```python
from build123d import *

# Parameters (mm, degrees)
F0_W          = 46
F0_H          = 58
F1_DEPTH      = 6
F2_W          = 38
F2_H          = 38
F3_DEPTH      = 3
F4_W          = 33
F4_H          = 33
F5_DEPTH      = 3.001
F6_W          = 26
F6_H          = 5
F7_DEPTH      = 3.001
F7_DEPTH_BACK = 3.001
F8_W          = 26
F8_H          = 5
F9_DEPTH      = 3.001
F9_DEPTH_BACK = 3.001
F10_SIZE      = 3
F11_W         = 4.5
F11_H         = 20
F12_DEPTH     = 46
F13_W         = 4
F13_H         = 9.5
F14_DEPTH     = 10
F15_T4_DEPTH  = 4
F16_W         = 4
F16_H         = 9.5
F17_DEPTH     = 10
F18_T4_DEPTH  = 4
F19_R         = 2
F20_DEPTH     = 4.501


# Not quite as in the source:
# - a fillet or chamfer that OpenCascade refuses, or shapes differently, is made with other operations: its cross-section is extruded or revolved along the edge and cut away or added


with BuildPart() as f1:
    # F0 (on Top) → F1 (new body)
    with BuildSketch(Plane.XY):
        Rectangle(F0_W, F0_H)
    extrude(amount=F1_DEPTH)

    # F2 (on face) → F3 (cut)
    with BuildSketch(Plane.XY.offset(6)):
        with Locations((0, 4)):
            Rectangle(F2_W, F2_H)
    extrude(amount=-F3_DEPTH, mode=Mode.SUBTRACT)

    # F4 (on face) → F5 (cut, through all)
    with BuildSketch(Plane.XY.offset(3)):
        with Locations((0, 4)):
            Rectangle(F4_W, F4_H)
    extrude(amount=-F5_DEPTH, mode=Mode.SUBTRACT)

    # F6 (on face) → F7 (cut, two sides)
    with BuildSketch(Plane.XY.offset(3)) as f7_sk:
        with Locations((0, 23)):
            Rectangle(F6_W, F6_H)
    extrude(amount=-F7_DEPTH, mode=Mode.SUBTRACT)
    extrude(f7_sk.sketch, amount=F7_DEPTH_BACK, mode=Mode.SUBTRACT)

    # F8 (on face) → F9 (cut, two sides)
    with BuildSketch(Plane.XY.offset(3)) as f9_sk:
        with Locations((0, -15)):
            Rectangle(F8_W, F8_H)
    extrude(amount=F9_DEPTH, mode=Mode.SUBTRACT)
    extrude(f9_sk.sketch, amount=-F9_DEPTH_BACK, mode=Mode.SUBTRACT)

    # F10
    f10_edges = [f1.edges().sort_by_distance(p)[0] for p in [
        (-13, -12.5, 1.5),
        (-13, 20.5, 1.5),
        (13, 20.5, 1.5),
        (13, -12.5, 1.5),
    ]]
    chamfer(f10_edges, length=F10_SIZE)

    # F11 (on face) → F12 (join)
    with BuildSketch(Plane(origin=(-23, 0, 0), x_dir=(0, -1, 0), z_dir=(-1, 0, 0))):
        with Locations((26.75, 10)):
            Rectangle(F11_W, F11_H)
    extrude(amount=-F12_DEPTH)

    # F13 (on face) → F14 (join)
    with BuildSketch(Plane.XY.offset(6)):
        with Locations((-21, -19.75)):
            Rectangle(F13_W, F13_H)
    extrude(amount=F14_DEPTH)

    # F15: chamfer of 10 on 1 edges, made by hand


with BuildPart() as f15_tool2:
    # F15_s3 → F15_t4 (new body)
    with BuildSketch(Plane.YZ.offset(-19)):
        with BuildLine():
            Line((-14.7171572875, 5.7171572875), (-25.2828427125, 16.2828427125))
            Line((-25.2828427125, 16.2828427125), (-25.2828427125, 16.4828427125))
            ThreePointArc((-25.2828427125, 16.4828427125), (-20.1414213562, 16.2), (-15, 16.2))
            Line((-15, 16.2), (-14.8, 16))
            ThreePointArc((-14.8, 16), (-14.8, 10.8585786438), (-14.5171572875, 5.7171572875))
            Line((-14.5171572875, 5.7171572875), (-14.7171572875, 5.7171572875))
        make_face()
    extrude(amount=-F15_T4_DEPTH)

    split(bisect_by=Plane.XY.offset(6), keep=Keep.TOP)

    split(bisect_by=Plane.XZ.offset(24.5), keep=Keep.BOTTOM)


with BuildPart() as f1_1:
    add(f1.part)

    # F15_t1: cut F15_tool2
    add(f15_tool2.part, mode=Mode.SUBTRACT)

    # F16 (on face) → F17 (join)
    with BuildSketch(Plane.XY.offset(6)):
        with Locations((21, -19.75)):
            Rectangle(F16_W, F16_H)
    extrude(amount=F17_DEPTH)

    # F18: chamfer of 10 on 1 edges, made by hand


with BuildPart() as f18_tool2:
    # F18_s3 → F18_t4 (new body)
    with BuildSketch(Plane.YZ.offset(23)):
        with BuildLine():
            Line((-14.7171572875, 5.7171572875), (-25.2828427125, 16.2828427125))
            Line((-25.2828427125, 16.2828427125), (-25.2828427125, 16.4828427125))
            ThreePointArc((-25.2828427125, 16.4828427125), (-20.1414213562, 16.2), (-15, 16.2))
            Line((-15, 16.2), (-14.8, 16))
            ThreePointArc((-14.8, 16), (-14.8, 10.8585786438), (-14.5171572875, 5.7171572875))
            Line((-14.5171572875, 5.7171572875), (-14.7171572875, 5.7171572875))
        make_face()
    extrude(amount=-F18_T4_DEPTH)

    split(bisect_by=Plane.XY.offset(6), keep=Keep.TOP)

    split(bisect_by=Plane.XZ.offset(24.5), keep=Keep.BOTTOM)


with BuildPart() as f1_2:
    add(f1_1.part)

    # F18_t1: cut F18_tool2
    add(f18_tool2.part, mode=Mode.SUBTRACT)

    # F19 (on face) → F20 (cut, through all)
    with BuildSketch(Plane(origin=(0, -24.5, 0), x_dir=(-1, 0, 0), z_dir=(0, 1, 0))):
        with Locations((11, 14)):
            Circle(F19_R)
        with Locations((-11, 14)):
            Circle(F19_R)
    extrude(amount=-F20_DEPTH, mode=Mode.SUBTRACT)


solid = f1_2.part
```
Check sheet for the modelled part. Datum: model origin and axes. Units: mm. A direction names the side the tool comes from. Coordinates: 2 decimals unless noted, no trailing zeros. Loops run counter-clockwise (first coordinate to the right, second up) from the corner with the lowest first, then second, coordinate; pieces in that order, holes last.
1) Access from +Z, -Z, +X, -X, +Y, -Y to the whole of each face (thin tool, end or side, straight path). Record for faces 5 (the face through (0, -17.5, 3)), 6 (the face through (0, 28, 6)), 7 (the face through (16, 23, 5)), 8 (the face through (19, -21, 10)).
2) Material ranges on probe 1 along X at (y, z) = (-11, 5.25); probe 2 along Z at (x, y) = (-11, -28.1); probe 3 along Y at (x, z) = (3, 1), recorded low to high.
3) Sectioned sample at A-A (z = 14). Record the boundary of the cut face in (x, y).
4) Sectioned sample at B-B (x = -3). Record the boundary of the cut face in (y, z).
5) Release check for a two-part mould opening along Y. For faces 1 (the face through (0, 25.5, 3)), 2 (the face through (0, -19, 0)), 3 (the face through (21, -20, 11)), 4 (the face through (-14.1, -14.4, 1.7)) record: released by +Y, released by -Y, zero draft, split by the parting line, or undercut.
6) Gauge pin test, flat end, axial feed: pin 1 (22 mm diameter, centred on x = -10.5, y = 14, fed in from +Z). Record the tip position at first contact, or that the pin passes through.
7) Sectioned sample at C-C (y = 7). Record the boundary of the cut face in (x, z).
8) Sectioned sample at D-D (x = 11). Record the boundary of the cut face in (y, z), and give its area (3 significant figures).
Check sheet entries:
1. face 5: +Z, -Z
1. face 6: +Z, +X, -X, +Y
1. face 7: +Z
1. face 8: +Z, +Y
2. probe 1: x = -23 to -19, 19 to 23
2. probe 2: z = 0 to 12, 16 to 20
2. probe 3: y = -29 to -17.5, 25.5 to 29
3. outline: (-23, -29) - (-13, -29) - (-13, -24.5) - (-19, -24.5) - (-19, -23) - (-23, -23) - close; (-9, -29) - (9, -29) - (9, -24.5) - (-9, -24.5) - close; (13, -29) - (23, -29) - (23, -23) - (19, -23) - (19, -24.5) - (13, -24.5) - close
4. outline: (-29, 0) - (-17.5, 0) - (-17.5, 6) - (-24.5, 6) - (-24.5, 20) - (-29, 20) - close; (25.5, 0) - (29, 0) - (29, 6) - (25.5, 6) - close
5. face 1: undercut
5. face 2: zero draft
5. face 3: released by +Y
5. face 4: undercut
6. pin 1: stops at z = 6
7. outline: (-23, 0) - (-16.5, 0) - (-16.5, 3) - (-19, 3) - (-19, 6) - (-23, 6) - close; (16.5, 0) - (23, 0) - (23, 6) - (19, 6) - (19, 3) - (16.5, 3) - close
8. outline: (-29, 0) - (-17.5, 0) - (-17.5, 6) - (-24.5, 6) - (-24.5, 12) - (-29, 12) - close; (-29, 16) - (-24.5, 16) - (-24.5, 20) - (-29, 20) - close; (25.5, 0) - (29, 0) - (29, 6) - (25.5, 6) - close
8. area: 135 mm2
